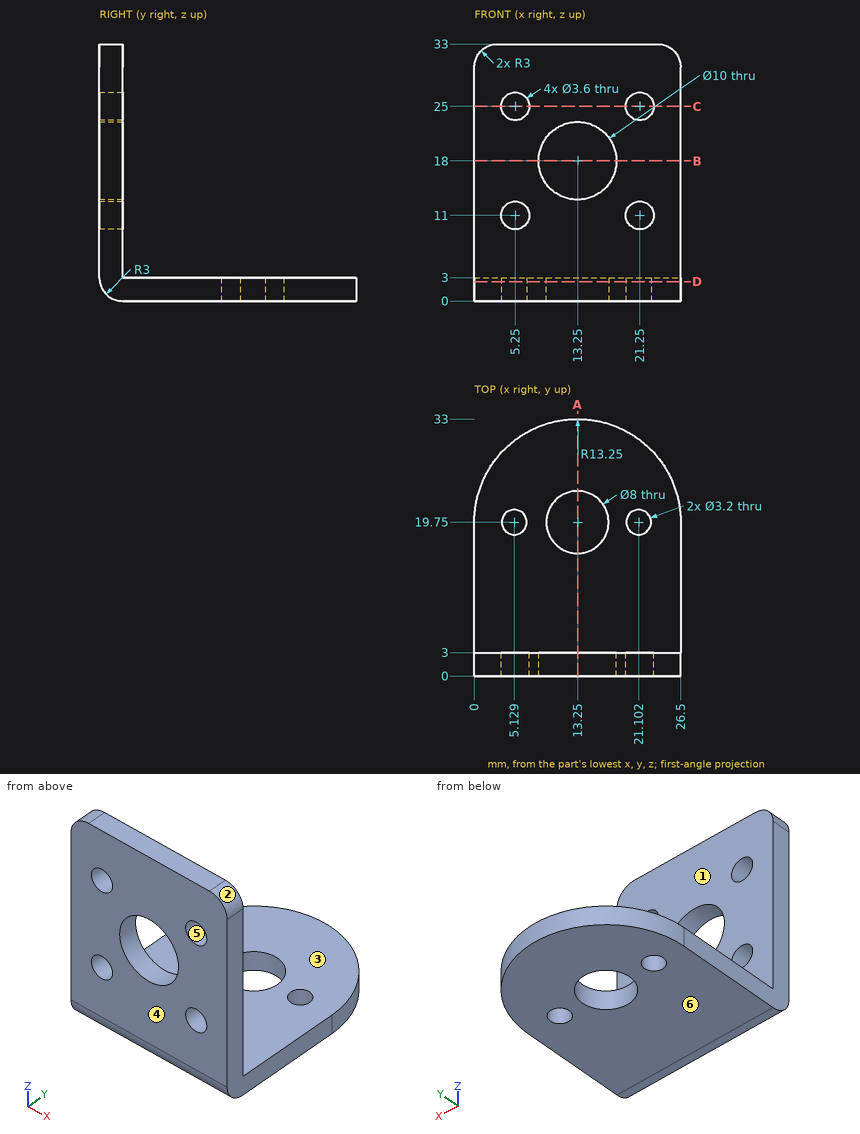
Geometry: see drawing. Coordinates: mm, zero at the bounding-box minimum. A direction names the side the tool comes from. Give positions to 0.01 mm unless a question says otherwise; leave off trailing zeros. Loops run counter-clockwise (first coordinate to the right, second up) from the corner with the lowest first, then second, coordinate; pieces in that order, holes last. Notation, with made-up numbers: (78, -6) -> (82, -6) arc R23 ccw to (82, 6) -> close; hole circle Ø9 at (-29.5, -7.75). An arc over 180 degrees is marked (long way). Answer as a JSON object with one key per item and string values. Group by question number.
Item 1: Cut plane C-C, the plane z = 25. Return the cut outline in (x, y), and give its area (3 significant figures).
Item 2: Reachability of the marked faces 1 and 2 from +Z, -Z, +X, -X, +Y, -Y: full face, straight path, thin tool, end or side. Return the list, or none.
Item 3: Cut plane D-D, the plane z = 2.5. Return the cut outline in (x, y).
Item 4: Cut plane A-A, the plane x = 13.25. Return the cut outline in (y, z), and give its area (3 significant figures).
Item 5: Pull-direction query (Z, two-part tool) for the marked faces 3, 4, 5 and 6; classes: released by +Z, released by -Z, zero draft, split by the parting line, or undercut.
Item 6: Cut plane B-B, the plane z = 18. Return the cut outline in (x, y), and give its area (3 significant figures).
Item 7: Line query: probe 1 along X at (y, z) = (1.8, 25); probe 2 along X at (y, z) = (19, 1) (1 decimal); probe 3 along Z at (x, y) = (21.25, 1.05). Output: solid intervals per line, ascending.
Item 8: Pin query (flat end, axial travel): P1, Ø4, axis at x = 21.1, y = 19.75, coming from the +Z side; P2, Ø4, axis at x = 9.5, z = 3.5, coming from the +Y side; P3, Ø6, axis at x = 21.5, z = 23.5, coming from the +Y side. Return the tip coordinate at first contact, or that it passes through.
Checks:
{
 "1": {"outline": "(0, 0) -> (3.45, 0) -> (3.45, 3) -> (0, 3) -> close; (7.05, 0) -> (19.45, 0) -> (19.45, 3) -> (7.05, 3) -> close; (23.05, 0) -> (26.5, 0) -> (26.5, 3) -> (23.05, 3) -> close", "area": "57.9 mm²"},
 "2": {"face 1": "+Z, +X, -X, +Y", "face 2": "+Z, +X, +Y, -Y"},
 "3": {"outline": "(0, 0.04) -> (26.5, 0.04) -> (26.5, 19.75) arc R13.25 ccw to (0, 19.75) -> close; hole circle Ø3.2 at (5.13, 19.75); hole circle Ø8 at (13.25, 19.75); hole circle Ø3.2 at (21.1, 19.75)"},
 "4": {"outline": "(0, 3) arc R3 ccw to (3, 0) -> (15.75, 0) -> (15.75, 3) -> (3, 3) -> (3, 13) -> (0, 13) -> close; (0, 23) -> (3, 23) -> (3, 33) -> (0, 33) -> close; (23.75, 0) -> (33, 0) -> (33, 3) -> (23.75, 3) -> close", "area": "133 mm²"},
 "5": {"face 3": "released by +Z", "face 4": "zero draft", "face 5": "undercut", "face 6": "released by -Z"},
 "6": {"outline": "(0, 0) -> (8.25, 0) -> (8.25, 3) -> (0, 3) -> close; (18.25, 0) -> (26.5, 0) -> (26.5, 3) -> (18.25, 3) -> close", "area": "49.5 mm²"},
 "7": {"probe 1": "x = 0 to 3.45, 7.05 to 19.45, 23.05 to 26.5", "probe 2": "x = 0 to 3.7, 6.5 to 9.3, 17.2 to 19.7, 22.5 to 26.5", "probe 3": "z = 0.72 to 9.2, 12.8 to 23.2, 26.8 to 33"},
 "8": {"P1": "stops at z = 3", "P2": "stops at y = 32.88", "P3": "stops at y = 3"}
}
